from build123d import *


with BuildPart() as part:
    # Sketch1 → Revolve1 (revolve)
    with BuildSketch(Plane.XY, mode=Mode.PRIVATE) as revolve1_sk:
        with BuildLine():
            Line((-4.3688, 1.651), (3.104789807, 1.651))
            Line((3.104789807, 1.651), (4.3688, 2.6035))
            Line((4.3688, 2.6035), (4.3688, 3.0099))
            ThreePointArc((4.3688, 3.0099), (4.257207684, 3.279307684), (3.9878, 3.3909))
            Line((3.9878, 3.3909), (1.5748, 3.3909))
            ThreePointArc((1.5748, 3.3909), (1.305392316, 3.279307684), (1.1938, 3.0099))
            Line((1.1938, 3.0099), (1.1938, 2.1844))
            Line((1.1938, 2.1844), (-4.3688, 2.1844))
            Line((-4.3688, 2.1844), (-4.3688, 1.651))
        make_face()
    revolve(revolve1_sk.sketch.rotate(Axis((-4.3688, 0, 0), (1, 0, 0)), 90), axis=Axis((-4.3688, 0, 0), (1, 0, 0)))


solid = part.part
Geometry: final body of the model. Coordinates: model frame, mm. A direction names the side the tool comes from. Give positions to 0.01 mm unless a question says otherwise; leave off trailing zeros. Loops run counter-clockwise (first coordinate to the right, second up) from the corner with the lowest first, then second, coordinate; pieces in that order, holes last. Notation, with made-up numbers: M 23,29.5 L 81,29.5 A31 cw 81,61.5 Z; hole C 5.25,29.5 d9. An arc over 180 degrees is marked long. Put each result on its own line as item: value. Start each with the question number.
1) Cut plane A-A (y = 0). Output: boundary loops of the cut face in (x, z), then the cut area to 3 significant figures.
2) Contact query for flat-ended pins moving along their axis: pin 1 (1.5 mm diameter, centred on x = 2.5, z = -0.5, fed in from -Y); pin 2 (2.5 mm diameter, centred on y = 0, z = 0, fed in from +X); pin 3 (2 mm diameter, centred on x = 3, z = 2, fed in from -Y); pin 4 (3 mm diameter, centred on x = -1, z = 1.5, fed in from -Y). Output: stop coordinate, or through.
3) Cut plane C-C (x = -3). Output: boundary loops of the cut face in (y, z), then the cut area to 3 significant figures.
4) Ray query, line 1 along Y through (x, z) = (-1.75, 0); line 2 along X through (y, z) = (2.25, -2); line 3 along Z through (x, y) = (1.5, 0.5). Return the intervals inside material, ascending.
5) Access query for faces 1 (the flat face through (4.369, -2, 2)), 2 (the cylindrical face through (-1.626, -0.656, 2.084)). Directions: +Z, -Z, +X, -X, +Y, -Y. A direction counts if a zero-diameter tool reaches every point of the face in a straight line with its end or side. Return the directions, or none.
6) Pull-direction query (Z, two-part tool) for faces 3 (the flat face through (-4.369, -2, 0)), 4 (the cylindrical face through (-0.58, -0.496, 1.575)), 5 (the cylindrical face through (2.764, -1.019, 3.234)); classes: pulls with the +Z half, pulls with the -Z half, needs draft (parallel to the pull), parting line crosses it, or undercut.
Verdict:
1. outline: M -4.37,-2.18 L 1.19,-2.18 L 1.19,-3.01 A0.38 ccw 1.57,-3.39 L 3.99,-3.39 A0.38 ccw 4.37,-3.01 L 4.37,-2.6 L 3.1,-1.65 L -4.37,-1.65 Z; M -4.37,1.65 L 3.1,1.65 L 4.37,2.6 L 4.37,3.01 A0.38 ccw 3.99,3.39 L 1.57,3.39 A0.38 ccw 1.19,3.01 L 1.19,2.18 L -4.37,2.18 Z
1. area: 15.7 mm2
2. pin 1: y = -3.39
2. pin 2: through
2. pin 3: y = -3.24
2. pin 4: y = -2.18
3. outline: C 0,0 d4.37; hole C 0,0 d3.3
3. area: 6.43 mm2
4. line 1: -2.18 to -1.65, 1.65 to 2.18
4. line 2: 1.19 to 4.37
4. line 3: -3.35 to -1.57, 1.57 to 3.35
5. face 1: +Z, -Z, +X, +Y, -Y
5. face 2: -X
6. face 3: needs draft
6. face 4: undercut
6. face 5: parting line crosses it
